Can you work these out from the model? Positions are in its coordinate system, mm. Face numbers are marked on the shaded views. A direction names the side the tool comes from. Round coordinates to 2 decimals unless told otherwise and drop trailing zeros. Write each loop counter-clockwise with the first axis right and the second up, starting at its lowest first coordinate (ties: lowest second). Pieces come first, ordered by that corner, then holes. Notation, with made-up numbers: (-33.5, 47) -> (-3.5, 47) arc R23 cw to (-3.5, 79) -> close; hole circle Ø1 at (-12, -23). An arc over 180 degrees is marked (long way). Write item = value, one per line. Start each with the question number.
1) If I drill on line 1 (X direction, y = 91, z = 18.5) (3 decimals); line 2 (Z direction, x = -9, y = 5.5) (3 decimals); line 3 (Y direction, x = -25.4, z = 2.35), over which ranges is the centre line in solid material (lowest first)?
2) For the marked faces 1 and 2, which set-ups out of +Z, -Z, +X, -X, +Y, -Y let a thin tool reach every point of the face, with its end or its side?
3) I'm going to push flat-ended pins straight in: pin 1 (6 mm diameter, centred on y = -10.5, z = 13.5, fed in from -X); pin 2 (17 mm diameter, centred on x = -25.4, y = 88.9, fed in from +Z); pin 3 (3.5 mm diameter, centred on x = -7, z = 23.5, fed in from -Y); pin 4 (1.6 mm diameter, centred on y = 26.5, z = 2, fed in from -X). Where does each tip first touch, or does it pass through?
4) Imagine slicing it at A-A, the plane z = 10.25. Please give me the cut outline in (x, y) (3 decimals), then the cut area to 3 significant figures.
5) Imagine slicing it at C-C, the plane x = -25.4. Please give me the cut outline in (y, z) (1 decimal), then the cut area to 3 significant figures.
6) Imagine slicing it at D-D, the plane y = 88.9. Please give me the cut outline in (x, z) (1 decimal), then the cut area to 3 significant figures.
7) Imagine slicing it at B-B, the plane y = 73. Please give me the cut outline in (x, z) (3 decimals).
8) Thinking about a two-plate mould opening in X: for the marked faces 3, 4 and 5, which applies, +X half, -X half, draft (parallel to the pull), parting line (faces both ways), or undercut?
Autodesk Inventor part; units mm, degrees
ref_plane "YZ Plane" through (0, 0, 0) normal (1, 0, 0) x (0, 1, 0)
ref_plane "XZ Plane" through (0, 0, 0) normal (0, 1, 0) x (-1, 0, 0)
ref_plane "XY Plane" through (0, 0, 0) normal (0, 0, 1) x (1, 0, 0)
sketch "Sketch1" plane through (0, 0, 0) normal (0, 1, 0) x (-1, 0, 0)
  line L0 (0, 0) -> (50.8, 0)
  line L1 (50.8, 0) -> (50.8, 25.4)
  line L2 (50.8, 25.4) -> (0, 25.4)
  line L3 (0, 25.4) -> (0, 0)
  line L4 (47.625, 3.175) -> (3.175, 3.175)
  line L5 (3.175, 3.175) -> (3.175, 22.225)
  line L6 (3.175, 22.225) -> (47.625, 22.225)
  line L7 (47.625, 22.225) -> (47.625, 3.175)
  dimension "d0" = 50.8
  dimension "d1" = 25.4
  dimension "d2" = 3.175
extrude "Extrusion1" add sketch "Sketch1" along normal blind 114.3
sketch "Sketch2" plane through (-50.8, 0, 25.4) normal (0, 0, 1) x (1, 0, 0)
  line L0 (0, 0) -> (38.1, 0)
  line L1 (38.1, 0) -> (38.1, 63.5)
  line L2 (38.1, 63.5) -> (0, 63.5)
  line L3 (0, 63.5) -> (0, 0)
  line L4 (0, 0) -> (50.8, 0)
  line L5 (0, 0) -> (0, 114.3)
  dimension "d5" = 38.1
  dimension "d6" = 63.5
extrude "Extrusion2" cut sketch "Sketch2" against normal blind 25.4
sketch "Sketch3" plane through (-50.8, 114.3, 25.4) normal (0, 0, 1) x (1, 0, 0)
  circle A0 centre (25.4, -25.4) radius 14.2875
  line L0 (0, 0) -> (50.8, 0)
  line L1 (0, -50.8) -> (0, 0)
  point P0 (50.8, -114.3)
  dimension "d9" = 28.575
  dimension "d10" = 25.4
  dimension "d11" = 25.4
extrude "Extrusion3" cut sketch "Sketch3" against normal blind 25.4
sketch "Sketch4" plane through (-50.8, 114.3, 25.4) normal (0, 0, 1) x (1, 0, 0)
  line L0 (50.8, -114.3) -> (59.4873, -138.1682)
  line L1 (47.4212, -114.3) -> (56.5038, -139.2541)
  line L2 (56.5038, -139.2541) -> (59.4873, -138.1682)
  line L3 (38.1, -114.3) -> (50.8, -114.3)
  line L4 (50.8, -114.3) -> (47.4212, -114.3)
  dimension "d14" = 25.4
  dimension "d15" = 3.175
  dimension "d16" = 110
extrude "Extrusion4" add sketch "Sketch4" against normal blind 25.4
properties part number "thumb block" material "Aluminum 6061"
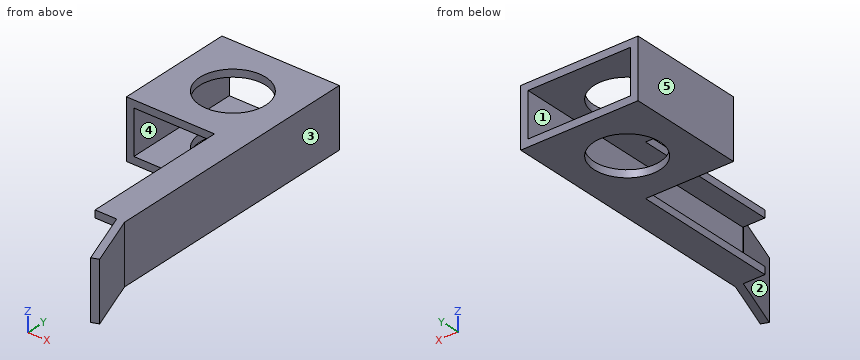
Reported:
q1.line_1 = -50.8 to -47.625, -3.175 to 0
q1.line_2 = 0 to 3.175, 22.225 to 25.4
q1.line_3 = 63.5 to 74.61, 103.19 to 114.3
q2.face_1 = +Y
q2.face_2 = +Z, -Z, -X, -Y
q3.pin_1 = -0.65
q3.pin_2 = through
q3.pin_3 = 0
q3.pin_4 = -12.7
q4.outline = (-50.8, 63.5) -> (-47.625, 63.5) -> (-47.625, 114.3) -> (-50.8, 114.3) -> close; (-3.379, 0) -> (5.704, -24.954) -> (8.687, -23.868) -> (0, 0) -> (0, 114.3) -> (-3.175, 114.3) -> (-3.175, 0) -> close
q4.area = 607 mm²
q5.outline = (63.5, 0) -> (74.6, 0) -> (74.6, 3.2) -> (63.5, 3.2) -> close; (63.5, 22.2) -> (74.6, 22.2) -> (74.6, 25.4) -> (63.5, 25.4) -> close; (103.2, 0) -> (114.3, 0) -> (114.3, 3.2) -> (103.2, 3.2) -> close; (103.2, 22.2) -> (114.3, 22.2) -> (114.3, 25.4) -> (103.2, 25.4) -> close
q5.area = 141 mm²
q6.outline = (-50.8, 0) -> (-39.7, 0) -> (-39.7, 3.2) -> (-47.6, 3.2) -> (-47.6, 22.2) -> (-39.7, 22.2) -> (-39.7, 25.4) -> (-50.8, 25.4) -> close; (-11.1, 0) -> (0, 0) -> (0, 25.4) -> (-11.1, 25.4) -> (-11.1, 22.2) -> (-3.2, 22.2) -> (-3.2, 3.2) -> (-11.1, 3.2) -> close
q6.area = 262 mm²
q7.outline = (-50.8, 0) -> (0, 0) -> (0, 25.4) -> (-50.8, 25.4) -> close; hole (-47.625, 3.175) -> (-3.175, 3.175) -> (-3.175, 22.225) -> (-47.625, 22.225) -> close
q8.face_3 = +X half
q8.face_4 = undercut
q8.face_5 = -X half
